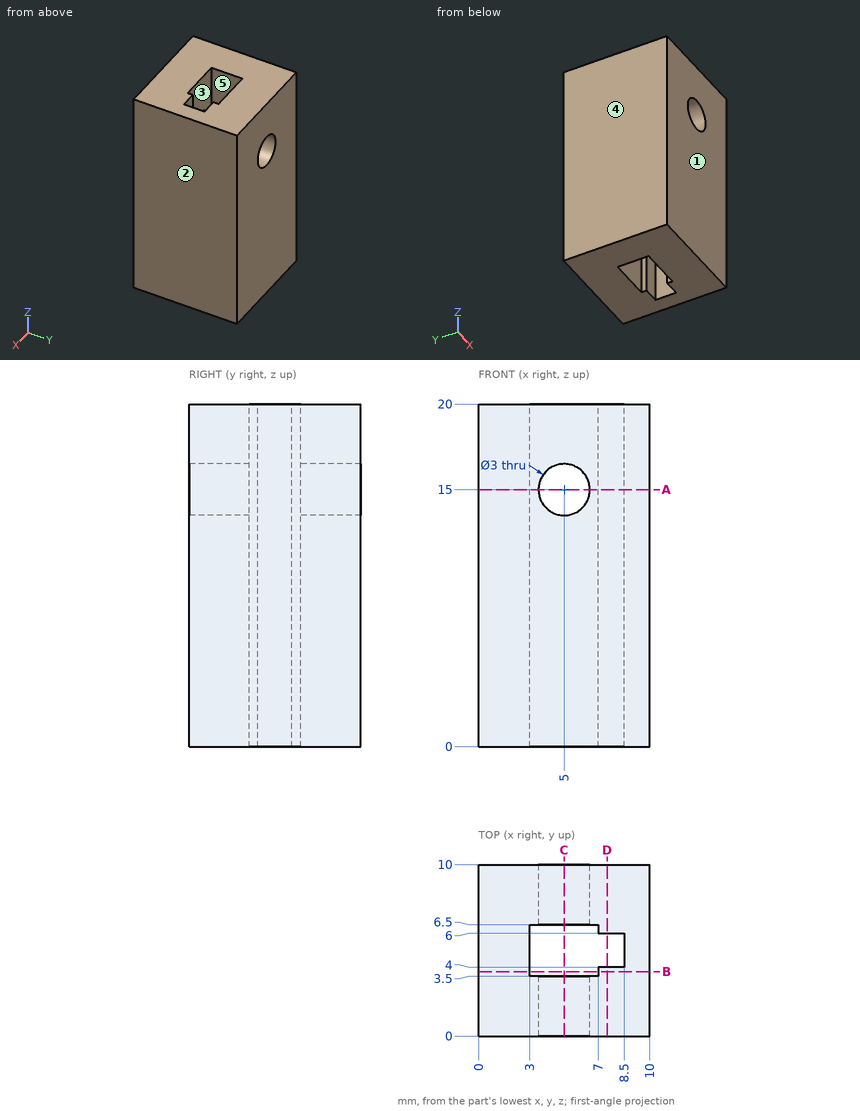
Could you check a few things on this drawing? It's one solid part, dimensions in mm from its lowest x, y, z. A direction names the side the tool comes from. Give positions to 0.01 mm unless a question says otherwise; leave off trailing zeros. Order: outer loops, then holes, each group sorted by start corner. A loop starts at its lowest first (then second) coordinate and runs counter-clockwise, first axis right, second up. Notation, with made-up numbers: (35, 48) - (48, 48) arc R8 ccw to (48, 52) - close; hole circle Ø8 at (51.5, 16.25). An arc over 180 degrees is marked (long way). Return JSON: item names as keys, results as strings. Group by question number.
Q1. Suppose I cut it at A-A, the plane z = 15. Please give me the cut outline in (x, y).
Q2. Suppose I cut it at C-C, the plane x = 5. Please give me the cut outline in (y, z).
Q3. Will this pin go through, and if not, where does the flat tip stop? pin 1 Ø2.5 at (x, z) = (5, 15) entering from -Y.
Q4. Suppose I cut it at D-D, the plane x = 7.5. Please give me the cut outline in (y, z).
Q5. Suppose I cut it at B-B, the plane y = 3.75. Please give me the cut outline in (x, z).
Q6. Please list where these lines run through material, in increasing order: line 1 along Y through (x, z) = (6.5, 2.25); line 2 along Z through (x, y) = (5, 8.7); line 3 along X through (y, z) = (4.25, 10.5). Write a range as [from, to].
Q7. Thinking about a two-plate mould opening in Y: for the marked faces 1, 2 and 3, which applies, pulls with the +Y half, pulls with the -Y half, needs draft (parallel to the pull), parting line crosses it, or undercut?
Q8. Which directions (+Z, -Z, +X, -X, +Y, -Y) give clear straight access to the entire face, cutting with the end or side of a thin tool? Please do the marked faces 4 and 5.
Resolved:
{
 "1": {"outline": "(0, 0) - (3.5, 0) - (3.5, 3.5) - (3, 3.5) - (3, 6.5) - (3.5, 6.5) - (3.5, 10) - (0, 10) - close; (6.5, 0) - (10, 0) - (10, 10) - (6.5, 10) - (6.5, 6.5) - (7, 6.5) - (7, 6) - (8.5, 6) - (8.5, 4) - (7, 4) - (7, 3.5) - (6.5, 3.5) - close"},
 "2": {"outline": "(0, 0) - (3.5, 0) - (3.5, 13.5) - (0, 13.5) - close; (0, 16.5) - (3.5, 16.5) - (3.5, 20) - (0, 20) - close; (6.5, 0) - (10, 0) - (10, 13.5) - (6.5, 13.5) - close; (6.5, 16.5) - (10, 16.5) - (10, 20) - (6.5, 20) - close"},
 "3": {"pin 1": "passes through"},
 "4": {"outline": "(0, 0) - (4, 0) - (4, 20) - (0, 20) - close; (6, 0) - (10, 0) - (10, 20) - (6, 20) - close"},
 "5": {"outline": "(0, 0) - (3, 0) - (3, 20) - (0, 20) - close; (7, 0) - (10, 0) - (10, 20) - (7, 20) - close"},
 "6": {"line 1": "y = [0, 3.5], [6.5, 10]", "line 2": "z = [0, 13.5], [16.5, 20]", "line 3": "x = [0, 3], [8.5, 10]"},
 "7": {"face 1": "pulls with the -Y half", "face 2": "needs draft", "face 3": "undercut"},
 "8": {"face 4": "+Z, -Z, -X, +Y, -Y", "face 5": "+Z, -Z"}
}
